Read the model definition and answer for the solid it produces. Units are mm, in the model's axes. A direction names the side the tool comes from. Coordinates: 2 decimals unless noted, no trailing zeros. Order: outer loops, then holes, each group sorted by start corner. A loop starts at its lowest first (then second) coordinate and runs counter-clockwise, first axis right, second up. Notation, with made-up numbers: (-17, -21) - (42, -21) arc R16 cw to (42, -10) - close; hole circle Ø3 at (60.25, 36.5). An arc over 180 degrees is marked (long way). Use one line per item in the form item = value.
```python
from build123d import *

# Parameters (mm, degrees)
ESBO_O2_R             = 12.7
CORTE_EXTRUS_O1_DEPTH = 102.6
PADR_OCIRCULAR1_COUNT = 8


with BuildPart() as part:
    # Esboço1 → Revolução1 (revolve)
    with BuildSketch(Plane.XY):
        Polygon((48.59, 0), (48.59, 107.95), (78.615, 107.95), (78.615, 101.6), (136.525, 101.6), (136.525, 63.5), (76.2, 63.5), (57.15, 12.29), (57.15, 0), align=None)
    revolve(axis=Axis((0, 0, 0), (0, 1, 0)))

    # Esboço2 → Corte-extrusão1 (cut, through all)
    with BuildSketch(Plane(origin=(0, 101.6, 0), x_dir=(1, 0, 0), z_dir=(0, 1, 0))):
        with Locations((41.310676524, 99.732795535)):
            Circle(ESBO_O2_R)
    corte_extrus_o1 = extrude(amount=-CORTE_EXTRUS_O1_DEPTH, mode=Mode.SUBTRACT)

    # PadrãoCircular1: Corte-extrusão1 ×8 about axis
    padr_ocircular1_axis = Axis((0, 0, 0), (0, 1, 0))
    for i in range(1, PADR_OCIRCULAR1_COUNT):
        add(corte_extrus_o1.rotate(padr_ocircular1_axis, i * 360 / PADR_OCIRCULAR1_COUNT), mode=Mode.SUBTRACT)


solid = part.part
```
(1) Straight lines are drawn through the part: L1, parallel to X at y = 83, z = 40; L2, parallel to X at y = 94, z = -103.5; L3, parallel to Z at x = 38, y = 70.5. For each, find the intervals that lie inside material, in ascending order.
Answer list:
L1 = -130.53 to -112.36, -87.1 to -27.59, 27.59 to 87.1, 112.36 to 130.53
L2 = -89.03 to -53.44, -29.18 to 29.18, 53.44 to 89.03
L3 = -131.13 to -111.99, -87.47 to -30.28, 30.28 to 87.47, 111.99 to 131.13
(2) Section C-C, the plane y = 97 is taken. State how many separate pieces and enclosed holes the cut face has, then the cut area to 3 significant figures.
Answer list:
separate_pieces = 1
enclosed_holes = 9
area = 47,100 mm2
(3) Given pin 1 Ø1.5 at (x, y) = (105, 86) entering from +Z; pin 2 Ø12 at (x, y) = (94.5, 96) entering from +Z; pin 3 Ø5 at (x, z) = (86, 103) entering from +Y, each flat-ended and moving along its own axis, determine where each tip first touches the part or whether it passes through.
Answer list:
pin_1 = 88.15
pin_2 = 103.96
pin_3 = 101.6
(4) Section B-B, the plane x = 0 is taken. Write down the section's boundary in (y, z) (3 decimals).
Answer list:
outline = (0, -57.15) - (12.29, -57.15) - (63.5, -76.2) - (63.5, -136.525) - (101.6, -136.525) - (101.6, -78.615) - (107.95, -78.615) - (107.95, -48.59) - (0, -48.59) - close; (0, 48.59) - (107.95, 48.59) - (107.95, 78.615) - (101.6, 78.615) - (101.6, 136.525) - (63.5, 136.525) - (63.5, 76.2) - (12.29, 57.15) - (0, 57.15) - close
(5) Which of the six approach directions +Z, -Z, +X, -X, +Y, -Y give full straight-line access (tool end or side, diameter ignored) to faces 4 (the cylindrical face through (-39.657, 82.817, 112.325)), 5 (the cylindrical face through (-17.042, 104.731, 76.746))?
Answer list:
face_4 = +Y, -Y
face_5 = +Y
(6) Section A-A, the plane z = 0 is taken. Write down the section's boundary in (x, y) (3 decimals), then the cut area to 3 significant figures.
Answer list:
outline = (-136.525, 63.5) - (-76.2, 63.5) - (-57.15, 12.29) - (-57.15, 0) - (-48.59, 0) - (-48.59, 107.95) - (-78.615, 107.95) - (-78.615, 101.6) - (-136.525, 101.6) - close; (48.59, 0) - (57.15, 0) - (57.15, 12.29) - (76.2, 63.5) - (136.525, 63.5) - (136.525, 101.6) - (78.615, 101.6) - (78.615, 107.95) - (48.59, 107.95) - close
area = 9,140 mm2
(7) The mould has two halves that part along X. Classify faces 1 (the flat face through (59, 63.5, 59)), 2 (the cylindrical face through (35.443, 82.817, 110.996)), 3 (the cylindrical face through (-57.095, 6.059, -2.513)): +X half, -X half, draft (parallel to the pull), parting line (faces both ways), or undercut.
Answer list:
face_1 = draft
face_2 = undercut
face_3 = parting line
(8) Section D-D, the plane x = -104 is taken. Write down the section's boundary in (y, z), then the cut area to 3 significant figures.
Answer list:
outline = (63.5, -88.45) - (101.6, -88.45) - (101.6, -53.27) - (63.5, -53.27) - close; (63.5, -29.35) - (101.6, -29.35) - (101.6, 29.35) - (63.5, 29.35) - close; (63.5, 53.27) - (101.6, 53.27) - (101.6, 88.45) - (63.5, 88.45) - close
area = 4,920 mm2
